Here's how the part is built. I have some questions about the finished solid (model axes, mm). Face numbers are marked on the shaded views. A direction names the side the tool comes from. Give positions to 0.01 mm unless a question says otherwise; leave off trailing zeros. Order: outer loops, then holes, each group sorted by start corner. A loop starts at its lowest first (then second) coordinate and runs counter-clockwise, first axis right, second up. Notation, with made-up numbers: M -35,-0.5 L -20,-0.5 A10 cw -20,14.5 Z; hole C 84,-10 d6. An arc over 180 degrees is marked long. Use one line per item in the form item = value.
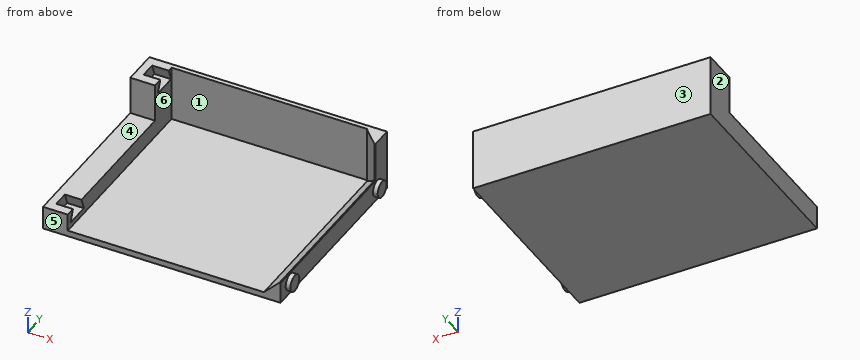
Autodesk Inventor part; units mm, degrees
ref_plane "YZ Plane" through (0, 0, 0) normal (1, 0, 0) x (0, 1, 0)
ref_plane "XZ Plane" through (0, 0, 0) normal (0, 1, 0) x (-1, 0, 0)
ref_plane "XY Plane" through (0, 0, 0) normal (0, 0, 1) x (1, 0, 0)
sketch "Skizze1" plane through (0, 0, 0) normal (1, 0, 0) x (0, 1, 0)
  line L0 (12.7735, 187.5054) -> (12.7735, 177.5054) construction
  line L1 (12.7735, 177.5054) -> (95.7735, 177.5054) construction
  line L2 (95.7735, 177.5054) -> (95.7735, 203.5054) construction
  line L3 (91.4537, 203.5054) -> (93.2735, 198.5054) construction
  line L4 (95.7735, 203.5054) -> (80.7735, 203.5054) construction
  line L5 (93.2735, 198.5054) -> (83.2735, 198.5054) construction
  line L6 (83.2735, 198.5054) -> (85.0934, 203.5054) construction
  line L7 (80.7735, 203.5054) -> (80.7735, 187.5054) construction
  line L8 (80.7735, 187.5054) -> (12.7735, 187.5054) construction
  line L9 (12.7735, 187.5054) -> (12.7735, 177.5054) construction
  line L10 (15.2735, 182.5054) -> (17.0934, 187.5054) construction
  line L11 (25.2735, 182.5054) -> (15.2735, 182.5054) construction
  line L12 (23.4537, 187.5054) -> (25.2735, 182.5054) construction
  line L13 (95.7735, 177.5054) -> (95.7735, 203.3054)
  line L14 (95.7735, 203.3054) -> (91.5797, 203.3054)
  line L15 (91.5797, 203.3054) -> (93.3995, 198.3054)
  line L16 (93.3995, 198.3054) -> (83.1475, 198.3054)
  line L17 (83.1475, 198.3054) -> (84.9674, 203.3054)
  line L18 (84.9674, 203.3054) -> (80.8735, 203.3054)
  line L19 (80.8735, 203.3054) -> (80.8735, 187.3054)
  line L20 (80.8735, 187.3054) -> (23.6329, 187.3054)
  line L21 (23.6329, 187.3054) -> (25.4527, 182.3054)
  line L22 (25.4527, 182.3054) -> (15.0943, 182.3054)
  line L23 (15.0943, 182.3054) -> (16.9142, 187.3054)
  line L24 (16.9142, 187.3054) -> (12.8735, 187.3054)
  line L25 (12.8735, 187.3054) -> (12.8735, 177.5054)
  line L26 (12.8735, 177.5054) -> (95.7735, 177.5054)
  point P0 (0, 0)
  dimension "d0" = 0.2
  dimension "d1" = 0.05
  dimension "d2" = 0.05
  dimension "d3" = 0.1
  dimension "d4" = 0.2
  dimension "d5" = 0.1
  dimension "d6" = 0.1
  dimension "d7" = 0.1
extrude "Extrusion1" add sketch "Skizze1" along normal blind 7
sketch "Skizze2" plane through (0, 0, 0) normal (-1, 0, 0) x (0, 0, 1)
  line L0 (177.5054, 95.7735) -> (203.3054, 95.7735)
  line L1 (177.5054, 12.8735) -> (177.5054, 95.7735)
  line L2 (187.3054, 12.8735) -> (177.5054, 12.8735)
  line L3 (203.3054, 80.8735) -> (187.3054, 80.8735)
  line L4 (203.3054, 80.8735) -> (187.3054, 80.8735)
  line L5 (187.3054, 12.8735) -> (187.3054, 80.8735)
  line L6 (187.3054, 80.8735) -> (203.3054, 80.8735)
  line L7 (203.3054, 95.7735) -> (203.3054, 91.5797)
  line L8 (203.3054, 80.8735) -> (203.3054, 95.7735)
  point P0 (0, 0)
extrude "Extrusion2" add sketch "Skizze2" along normal blind 3.4
sketch "Skizze3" plane through (7, 0, 0) normal (1, 0, 0) x (0, 0, -1)
  line L0 (-177.5054, 95.7735) -> (-203.3054, 95.7735)
  line L1 (-177.5054, 12.8735) -> (-177.5054, 95.7735)
  line L2 (-177.5054, 12.8735) -> (-180.0054, 12.8735)
  line L3 (-187.3054, 12.8735) -> (-177.5054, 12.8735)
  line L4 (-180.0054, 12.8735) -> (-180.0054, 93.7735)
  line L5 (-177.5054, 95.7735) -> (-177.5054, 12.8735)
  line L6 (-180.0054, 93.7735) -> (-203.3054, 93.7735)
  line L7 (-203.3054, 95.7735) -> (-203.3054, 91.5797)
  line L8 (-203.3054, 93.7735) -> (-203.3054, 95.7735)
  point P0 (0, 0)
  dimension "d12" = 2.5
  dimension "d13" = 2
  dimension "d14" = 2
extrude "Extrusion3" add sketch "Skizze3" along normal blind 89.5
sketch "Skizze4" plane through (96.5, 0, 0) normal (1, 0, 0) x (0, 0, -1)
  circle A0 centre (-182.5054, 20.2735) radius 3.5 construction
  circle A1 centre (-182.5054, 88.2735) radius 3.5 construction
  circle A2 centre (-182.5054, 20.2735) radius 3.45
  circle A3 centre (-182.5054, 88.2735) radius 3.45
  point P0 (0, 0)
  dimension "d17" = 0.05
  dimension "d18" = 0.05
extrude "Extrusion4" add sketch "Skizze4" along normal blind 2
sketch "Skizze5" plane through (96.5, 0, 0) normal (1, 0, 0) x (0, 0, -1)
  line L0 (-198.9754, 90.3435) -> (-183.0054, 90.3435) construction
  line L1 (-180.0054, 17.896) -> (-180.0054, 12.8735)
  circle A0 centre (-182.5054, 88.2735) radius 3.5 construction
  line L2 (-203.3054, 93.7735) -> (-180.0054, 93.7735)
  line L3 (-180.0054, 12.8735) -> (-186.5054, 12.8735)
  line L4 (-186.5054, 12.8735) -> (-186.5054, 93.7735)
  line L5 (-186.5054, 93.7735) -> (-180.0054, 93.7735)
  line L6 (-180.0054, 93.7735) -> (-180.0054, 12.8735)
  line L7 (-203.3054, 93.7735) -> (-186.5054, 93.7735)
  line L8 (-186.5054, 93.7735) -> (-186.5054, 86.7735)
  line L9 (-186.5054, 86.7735) -> (-203.3054, 86.7735)
  line L10 (-203.3054, 86.7735) -> (-203.3054, 93.7735)
  point P0 (0, 0)
  point P1 (-186.5054, 90.3435)
  dimension "d27" = 4
  dimension "d31" = 7
extrude "Extrusion5" add sketch "Skizze5" against normal blind 7
chamfer "Fase2" distance 6.5 angle 45 1 edges at (89.5, 49.8235, 186.5054)
chamfer "Fase3" distance 6.5 angle 45 1 edges at (89.5, 86.7735, 194.9054)
equation "\"d1\" = d2"
equation "\"d14\" = d13"
properties part number "Batcap3"
Q1. On a 3-axis mill with a long thin cutter (end or side, diameter ignored), from which of +Z, -Z, +X, -X, +Y, -Y can I reach the whole of each face in a straight line? I mean the marked faces 4, 5 and 6. Say none if no direction works.
Found:
face_4 = +Z, +X, -X, -Y
face_5 = +Z, -Z, +X, -X, -Y
face_6 = +Z, -Y
Q2. Thinking about a two-plate mould opening in X: for the marked faces 1, 2 and 3, which applies, +X half, -X half, draft (parallel to the pull), parting line (faces both ways), or undercut?
Found:
face_1 = undercut
face_2 = -X half
face_3 = draft
Q3. I want a section at A-A on z = 197. Write out the boundary of the cut face in (x, y).
Found:
outline = M -3.4,80.87 L 7,80.87 L 7,93.77 L 89.5,93.77 L 89.5,93.27 L 96,86.77 L 96.5,86.77 L 96.5,95.77 L -3.4,95.77 Z
Q4. I need wall thicknesses on L1, parallel to Z at x = 63.5, y = 72; L2, parallel to Y at x = 24.5, z = 193.5; L3, parallel to X at y = 84, z = 201.25. Which ranges of each line are inside material? Lowest first, please.
Found:
L1 = 177.51 to 180.01
L2 = 93.77 to 95.77
L3 = -3.4 to 7
Q5. I'm going to push flat-ended pins straight in: pin 1 Ø2 at (x, y) = (4, 88) entering from +Z; pin 2 Ø3 at (x, y) = (3.5, 62.5) entering from +Z; pin 3 Ø3.5 at (x, y) = (2.5, 20.5) entering from +Z. Where does each tip first touch, or does it pass through?
Found:
pin_1 = 198.31
pin_2 = 187.31
pin_3 = 182.31
Q6. I want a section at B-B on x = 12. Write out the boundary of the cut face in (y, z).
Found:
outline = M 12.87,177.51 L 95.77,177.51 L 95.77,203.31 L 93.77,203.31 L 93.77,180.01 L 12.87,180.01 Z
